from build123d import *

# Parameters (mm, degrees)
SKETCH1_W                         = 37.5
SKETCH1_H                         = 130
MOUNTING_PLATE_DEPTH              = 6.5
MOTOR_MOUNT_DEPTH                 = 10
LPATTERN1_COUNT                   = 2
LPATTERN1_PITCH                   = 30
LPATTERN1_COUNT_DIR2              = 2
LPATTERN1_PITCH_DIR2              = 30
MOTOR_HOLE_DEPTH                  = 7.5
LIMIT_SWITCH_PLACEMENT_DEPTH      = 1
LIMIT_SWITCH_PLACEMENT_DEPTH_BACK = 7.5
SKETCH8_R                         = 1.2
SLIDE_HOLES_DEPTH                 = 7.5
LPATTERN2_COUNT                   = 5
LPATTERN2_PITCH                   = 20
FILLET1_R                         = 5
SKETCH16_R                        = 2.5
CUT_EXTRUDE1_DEPTH                = 7.5
M3X0_5_TAPPED_HOLE1_D             = 2.5
M3X0_5_TAPPED_HOLE1_DEPTH         = 7.5
M3X0_5_TAPPED_HOLE1_TIP           = 0.751075774


with BuildPart() as part:
    # Sketch1 → Mounting Plate (new body)
    with BuildSketch(Plane.XY):
        with Locations((-18.75, 65)):
            Rectangle(SKETCH1_W, SKETCH1_H)
        with Locations((18.75, 65)):
            Rectangle(SKETCH1_W, SKETCH1_H)
    extrude(amount=MOUNTING_PLATE_DEPTH)

    # Sketch3 → Motor Mount (cut)
    with BuildSketch(Plane.XY.offset(6.5)):
        with BuildLine():
            Line((-2.5, 120), (-2.5, 125))
            ThreePointArc((-2.5, 125), (0.5, 128), (3.5, 125))
            Line((3.5, 125), (3.5, 120))
            ThreePointArc((3.5, 120), (0.5, 117), (-2.5, 120))
        make_face()
    motor_mount = extrude(amount=-MOTOR_MOUNT_DEPTH, mode=Mode.SUBTRACT)

    # LPattern1: Motor Mount 2 × 2
    with Locations(*[(i * LPATTERN1_PITCH, -j * LPATTERN1_PITCH_DIR2, 0) for i in range(LPATTERN1_COUNT) for j in range(LPATTERN1_COUNT_DIR2) if (i, j) != (0, 0)]):
        add(motor_mount, mode=Mode.SUBTRACT)

    # Sketch7 → Motor Hole (cut, through all)
    with BuildSketch(Plane.XY.offset(6.5)):
        with BuildLine():
            Line((4.5, 105), (4.5, 110))
            ThreePointArc((4.5, 110), (15.5, 121), (26.5, 110))
            Line((26.5, 110), (26.5, 105))
            ThreePointArc((26.5, 105), (15.5, 94), (4.5, 105))
        make_face()
    extrude(amount=-MOTOR_HOLE_DEPTH, mode=Mode.SUBTRACT)

    # Sketch2 → Limit Switch Placement (cut, two sides)
    with BuildSketch(Plane.XY.offset(6.5)) as limit_switch_placement_sk:
        with BuildLine():
            Line((-7.5, 415.136329844), (-7.5, 130))
            Line((-7.5, 130), (-7.5, 115))
            ThreePointArc((-7.5, 115), (-10.428932188, 107.928932188), (-17.5, 105))
            Line((-17.5, 105), (-37.5, 105))
            Line((-37.5, 105), (-322.636329844, 105))
            Line((-322.636329844, 105), (-722.642663203, 511.455212366))
            Line((-722.642663203, 511.455212366), (-407.50633336, 821.59154221))
            Line((-407.50633336, 821.59154221), (-7.5, 415.136329844))
        make_face()
    extrude(amount=LIMIT_SWITCH_PLACEMENT_DEPTH, mode=Mode.SUBTRACT)
    extrude(limit_switch_placement_sk.sketch, amount=-LIMIT_SWITCH_PLACEMENT_DEPTH_BACK, mode=Mode.SUBTRACT)

    # Sketch8 → Slide Holes (cut, through all)
    with BuildSketch(Plane.XY.offset(6.5)):
        with Locations((-17.5, 95)):
            Circle(SKETCH8_R)
    slide_holes = extrude(amount=-SLIDE_HOLES_DEPTH, mode=Mode.SUBTRACT)

    # LPattern2: Slide Holes ×5
    with Locations(*[(0, -i * LPATTERN2_PITCH, 0) for i in range(1, LPATTERN2_COUNT)]):
        add(slide_holes, mode=Mode.SUBTRACT)

    # Fillet1
    fillet1_edges = [part.edges().sort_by_distance(p)[0] for p in [
        (37.5, 130, 3.25),
        (37.5, 0, 3.25),
        (-37.5, 0, 3.25),
        (-7.5, 130, 3.25),
    ]]
    fillet(fillet1_edges, radius=FILLET1_R)

    # Sketch16 → Cut-Extrude1 (cut, through all)
    with BuildSketch(Plane.XY.offset(6.5)):
        with Locations((15.5, 9.71)):
            Circle(SKETCH16_R)
    extrude(amount=-CUT_EXTRUDE1_DEPTH, mode=Mode.SUBTRACT)

    # M3x0.5 Tapped Hole1
    with Locations(Plane(origin=(0, 0, 0), x_dir=(-1, 0, 0), z_dir=(0, -1, 0))):
        with Locations((-18.5, -3.25), (-12.5, -3.25)):
            Hole(M3X0_5_TAPPED_HOLE1_D / 2, depth=M3X0_5_TAPPED_HOLE1_DEPTH)
            with Locations((0, 0, -(M3X0_5_TAPPED_HOLE1_DEPTH + M3X0_5_TAPPED_HOLE1_TIP / 2))):  # 118° drill point
                Cone(0, M3X0_5_TAPPED_HOLE1_D / 2, M3X0_5_TAPPED_HOLE1_TIP, mode=Mode.SUBTRACT)


solid = part.part
The listing builds one solid part. Answer for the finished solid, in the listing's coordinates (mm). A direction names the side the tool comes from. Give positions to 0.01 mm unless a question says otherwise; leave off trailing zeros. Order: outer loops, then holes, each group sorted by start corner. A loop starts at its lowest first (then second) coordinate and runs counter-clockwise, first axis right, second up. Notation, with made-up numbers: (26.25, -23.5) - (38.25, -23.5) arc R16 ccw to (38.25, -9.5) - close; hole circle Ø10 at (-14, 86.25). An arc over 180 degrees is marked (long way). Use one line per item in the form item = value.
1) Find section B-B on x = 30.5. Determine the outline of the cut face in (y, z).
Verdict:
outline = (0, 0) - (87, 0) - (87, 6.5) - (0, 6.5) - close; (98, 0) - (117, 0) - (117, 6.5) - (98, 6.5) - close; (128, 0) - (130, 0) - (130, 6.5) - (128, 6.5) - close
2) Find section C-C on x = -25.5. Determine the outline of the cut face in (y, z), and give its area (4 significant figures).
Verdict:
outline = (0, 0) - (105, 0) - (105, 6.5) - (0, 6.5) - close
area = 682.5 mm^2
3) For faces 1 (the flat face through (-37.5, 54, 3)), 2 (the cylindrical face through (19.655, 3.802, 3.729)), 3 (the cylindrical face through (30.4, 98, 3.3)), determine the directions among +Z, -Z, +X, -X, +Y, -Y from which every point of the face is accessible in a straight line to the end or side of a thin tool.
Verdict:
face_1 = +Z, -Z, -X, +Y, -Y
face_2 = -Y
face_3 = +Z, -Z
4) The mould has two halves that part along Z. Classify faces 4 (the conical face through (12.5, 8.1, 3)), 5 (the flat face through (-1, 51, 0)), 6 (the cylindrical face through (-17.66, 56.19, 3.3)): released by +Z, released by -Z, zero draft, split by the parting line, or undercut.
Verdict:
face_4 = undercut
face_5 = released by -Z
face_6 = zero draft
5) Find section D-D on x = -14.5. Determine the outline of the cut face in (y, z), and give its area (3 significant figures).
Verdict:
outline = (0, 0) - (105.46, 0) - (105.46, 6.5) - (0, 6.5) - close
area = 685 mm^2
6) Each of these flat-tipped pins is pushed along its axis until it touches: pin 1 (3 mm diameter, centred on x = -25, z = 4, fed in from +Y); pin 2 (2 mm diameter, centred on y = 122, z = 4, fed in from -X). Where does it stop, or does it pass through?
Verdict:
pin_1 = 105
pin_2 = -7.5
7) Find section A-A on y = 9.71. Determine the outline of the cut face in (x, z).
Verdict:
outline = (-37.5, 0) - (13, 0) - (13, 6.5) - (-37.5, 6.5) - close; (18, 0) - (37.5, 0) - (37.5, 6.5) - (18, 6.5) - close
8) Consider probe 1 along Y at (x, z) = (15.5, 2.25); probe 2 along Y at (x, z) = (-17.5, 5); probe 3 along X at (y, z) = (93, 2). Determine where each line is inside the solid, lowest interval first. Write a range as [from, to].
Verdict:
probe_1 = [0, 7.21], [12.21, 94], [121, 130]
probe_2 = [0, 13.8], [16.2, 33.8], [36.2, 53.8], [56.2, 73.8], [76.2, 93.8], [96.2, 105]
probe_3 = [-37.5, -2.5], [3.5, 27.5], [33.5, 37.5]
